Design review of the part built by this model. Coordinates are the model's own, in mm. Face numbers are marked on the shaded views. A direction names the side the tool comes from. Give positions to 0.01 mm unless a question says otherwise; leave off trailing zeros. Write each loop counter-clockwise with the first axis right and the second up, starting at its lowest first coordinate (ties: lowest second). Pieces come first, ordered by that corner, then holes. Notation, with made-up numbers: M 42,58.5 L 69,58.5 A10 ccw 69,75.5 Z; hole C -36,-31.5 d8. An arc over 180 degrees is marked long. Answer in a Markdown table with one row per item.
```python
from build123d import *

# Parameters (mm, degrees)
F0_R     = 67.5
F1_DEPTH = 25
F3_DEPTH = 25.001
F4_R     = 5.25
F5_DEPTH = 25.001
F4_R_2   = 8
F6_DEPTH = 10


with BuildPart() as f1:
    # F0 (on Top) → F1 (new body)
    with BuildSketch(Plane.XY):
        Circle(F0_R)
    extrude(amount=F1_DEPTH)

    # F2 (on face) → F3 (cut, through all)
    with BuildSketch(Plane.XY.offset(25)):
        with BuildLine():
            ThreePointArc((-41.5, 0), (0, -41.5), (41.5, 0))
            ThreePointArc((41.5, 0), (0, 41.5), (-41.5, 0))
        make_face()
        with BuildLine():
            Line((41.5, -53.235327), (41.5, 0))
            ThreePointArc((41.5, 0), (0, -41.5), (-41.5, 0))
            Line((-41.5, 0), (-41.5, -53.235327))
            ThreePointArc((-41.5, -53.235327), (0, -67.5), (41.5, -53.235327))
        make_face()
    extrude(amount=-F3_DEPTH, mode=Mode.SUBTRACT)

    # F4 (on face) → F5 (cut, through all)
    with BuildSketch(Plane.XY.offset(25)):
        with Locations((51, -28)):
            Circle(F4_R)
        with Locations((-51, -28)):
            Circle(F4_R)
        with Locations((0, 58)):
            Circle(F4_R)
    extrude(amount=-F5_DEPTH, mode=Mode.SUBTRACT)

    # F4 (on face) → F6 (cut)
    with BuildSketch(Plane.XY.offset(25)):
        with Locations((51, -28)):
            Circle(F4_R_2)
        with Locations((51, -28)):
            Circle(F4_R, mode=Mode.SUBTRACT)
        with Locations((0, 58)):
            Circle(F4_R_2)
        with Locations((0, 58)):
            Circle(F4_R, mode=Mode.SUBTRACT)
        with Locations((-51, -28)):
            Circle(F4_R_2)
        with Locations((-51, -28)):
            Circle(F4_R, mode=Mode.SUBTRACT)
    extrude(amount=-F6_DEPTH, mode=Mode.SUBTRACT)


solid = f1.part
```
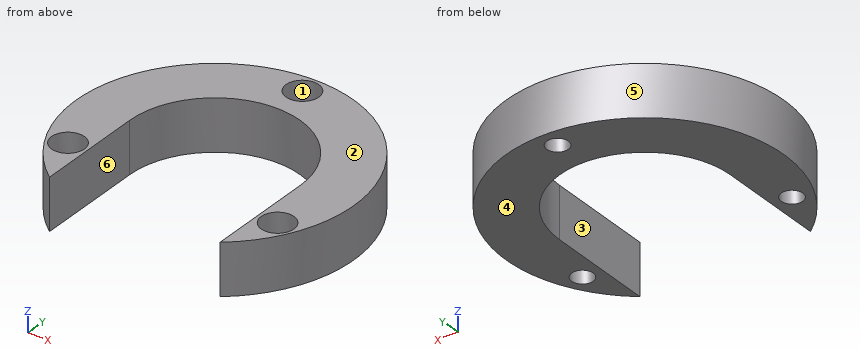
1) Add section A-A (z = 4.5). Write out the cut boundary in (x, y), and give its area (3 significant figures).
Geometry says:
| item | result |
|---|---|
| outline | M -41.5,-53.24 L -41.5,0 A41.5 cw 41.5,0 L 41.5,-53.24 A67.5 ccw long Z; hole C -51,-28 d10.5; hole C 0,58 d10.5; hole C 51,-28 d10.5 |
| area | 6,120 mm^2 |
2) For the marked faces 1, 2 and 3, list the 3-axis set-ups (+Z, -Z, +X, -X, +Y, -Y) from which the entire face can be reached by the end or side of a thin tool; tool diameter is ignored.
Geometry says:
| item | result |
|---|---|
| face 1 | +Z |
| face 2 | +Z, +X, -X, +Y, -Y |
| face 3 | +Z, -Z, -Y |
3) Insertion check: P1, Ø10, axis at x = -39.5, z = 4.5, coming from the +Y side; P2, Ø7.5, axis at y = -23.5, z = 9.5, coming from the -X side; P3, Ø8.5, axis at x = -51, y = -28, coming from the -Z side; P4, Ø10, axis at y = -7, z = 19, coming from the +X side. Each pin has a flat end and moves straight along its axis. Give the tip position at first contact, or say it passes through.
Geometry says:
| item | result |
|---|---|
| P1 | y = 58.02 |
| P2 | x = -64.55 |
| P3 | through |
| P4 | x = 67.47 |
4) Add section B-B (x = 51). Write out the cut boundary in (y, z), and give its area (3 significant figures).
Geometry says:
| item | result |
|---|---|
| outline | M -44.22,0 L -33.25,0 L -33.25,15 L -36,15 L -36,25 L -44.22,25 Z; M -22.75,0 L 44.22,0 L 44.22,25 L -20,25 L -20,15 L -22.75,15 Z |
| area | 1,890 mm^2 |
5) To check wall thickness, follow probe 1 along Y at (x, z) = (0, 6); probe 2 along X at (y, z) = (-26, 3.25); probe 3 along X at (y, z) = (-32.5, 6.75). State the ranges of each line that lie inside material, in increasing order. Write a range as [from, to].
Geometry says:
| item | result |
|---|---|
| probe 1 | [41.5, 52.75], [63.25, 67.5] |
| probe 2 | [-62.29, -55.85], [-46.15, -41.5], [41.5, 46.15], [55.85, 62.29] |
| probe 3 | [-59.16, -53.7], [-48.3, -41.5], [41.5, 48.3], [53.7, 59.16] |
6) Add section C-C (y = 58). Write out the cut boundary in (x, z).
Geometry says:
| item | result |
|---|---|
| outline | M -34.53,0 L -5.25,0 L -5.25,15 L -8,15 L -8,25 L -34.53,25 Z; M 5.25,0 L 34.53,0 L 34.53,25 L 8,25 L 8,15 L 5.25,15 Z |
7) The part is to be moulded in two halves that separate along X. For the marked faces 4, 5 and 6, say which applies: released by +X, released by -X, zero draft, split by the parting line, or undercut.
Geometry says:
| item | result |
|---|---|
| face 4 | zero draft |
| face 5 | split by the parting line |
| face 6 | undercut |
8) Add section D-D (y = -28). Write out the cut boundary in (x, z).
Geometry says:
| item | result |
|---|---|
| outline | M -61.42,0 L -56.25,0 L -56.25,15 L -59,15 L -59,25 L -61.42,25 Z; M -45.75,0 L -41.5,0 L -41.5,25 L -43,25 L -43,15 L -45.75,15 Z; M 41.5,0 L 45.75,0 L 45.75,15 L 43,15 L 43,25 L 41.5,25 Z; M 56.25,0 L 61.42,0 L 61.42,25 L 59,25 L 59,15 L 56.25,15 Z |
